Design review of the part built by this model. Coordinates are the model's own, in mm. Face numbers are marked on the shaded views. A direction names the side the tool comes from. Coordinates: 2 decimals unless noted, no trailing zeros. Write each loop counter-clockwise with the first axis right and the second up, starting at its lowest first coordinate (ties: lowest second). Pieces come first, ordered by that corner, then holes. Notation, with made-up numbers: (67, -27.75) -> (120, -27.75) arc R15 cw to (120, -22.75) -> close; hole circle Ø3 at (41, 48.5). An arc over 180 degrees is marked (long way). Return JSON: item names as keys, results as strings. Group by question number.
Autodesk Inventor part; units mm, degrees
ref_plane "FDT_PIRODACC_M1_XY" through (-9.9, 0, 0) normal (-1, 0, 0) x (0, 1, 0)
ref_plane "FDT_PIRODACC_M1_YZ" through (-9.9, 0, 0) normal (0, 1, 0) x (0, 0, -1)
ref_plane "FDT_PIRODACC_M1_ZX" through (-9.9, 0, 0) normal (0, 0, -1) x (-1, 0, 0)
sketch "Sketch_1" plane through (0, 0, 0) normal (0, 0, 1) x (1, 0, 0)
  line L0 (38, 0) -> (-4.2, 0)
  line L1 (-4.2, 0) -> (-4.2, 3)
  line L2 (-4.2, 3) -> (38, 3)
  line L3 (38, 3) -> (38, 0)
  line L4 (38, 0) -> (-4.2, 0)
revolve "Revolution1" add sketch "Sketch_1" angle 360 about axis through (38, 0, 0) along (1, 0, 0)
sketch "Sketch_11" plane through (0, 0, 0) normal (0, 0, 1) x (1, 0, 0)
  line L0 (38, 0) -> (35, 0)
  line L1 (35, 0) -> (35, 6)
  line L2 (35, 6) -> (38, 6)
  line L3 (38, 6) -> (38, 0)
  line L4 (38, 0) -> (35, 0)
revolve "Revolution2" add sketch "Sketch_11" angle 360 about axis through (38, 0, 0) along (1, 0, 0)
sketch "Sketch_19" plane through (0, 0, 0) normal (0, 0, 1) x (1, 0, 0)
  line L0 (-3.2, 0) -> (-14.2, 0)
  line L1 (-14.2, 0) -> (-14.2, 2.0095)
  line L2 (-14.2, 2.0095) -> (-13.7095, 2.5)
  line L3 (-13.7095, 2.5) -> (-6.7485, 2.5)
  line L4 (-6.7485, 2.5) -> (-5.1663, 1.9241)
  arc A0 (-5.1663, 1.9241) -> (-5.0295, 1.9) centre (-5.0295, 2.3) ccw
  line L5 (-5.0295, 1.9) -> (-4.6, 1.9)
  arc A1 (-4.6, 1.9) -> (-4.2, 2.3) centre (-4.6, 2.3) ccw
  line L6 (-4.2, 2.3) -> (-4.2, 2.5)
  line L7 (-4.2, 2.5) -> (-3.2, 2.5)
  line L8 (-3.2, 2.5) -> (-3.2, 0)
  line L9 (-3.2, 0) -> (-14.2, 0)
revolve "Revolution3" add sketch "Sketch_19" angle 360 about axis through (-3.2, 0, 0) along (1, 0, 0)
thread "Thread1"
sketch "Sketch_20" plane through (0, 0, 0) normal (0, 0, 1) x (1, 0, 0)
  line L0 (-23.4, -10.5) -> (3.1188, -10.5)
  line L1 (3.1188, -10.5) -> (-1.5, -2.5)
  line L2 (-1.5, -2.5) -> (-4.2, -2.5)
  line L3 (-4.2, -2.5) -> (-4.2, -7.5)
  line L4 (-4.2, -7.5) -> (-19.2, -7.5)
  line L5 (-19.2, -7.5) -> (-19.2, 7.5)
  line L6 (-19.2, 7.5) -> (-4.2, 7.5)
  line L7 (-4.2, 7.5) -> (-4.2, 2.5)
  line L8 (-4.2, 2.5) -> (-1.5, 2.5)
  line L9 (-1.5, 2.5) -> (3.1188, 10.5)
  line L10 (3.1188, 10.5) -> (-23.4, 10.5)
  line L11 (-23.4, 10.5) -> (-23.4, -10.5)
extrude "Extrusion1" cut sketch "Sketch_20" along normal mid plane 12
ref_plane "FDT_PIRODACC_M1_XY" through (-9.9, 0, 0) normal (-1, 0, 0) x (0, 1, 0)
ref_plane "FDT_PIRODACC_M1_YZ" through (-9.9, 0, 0) normal (0, 1, 0) x (0, 0, -1)
ref_plane "FDT_PIRODACC_M1_ZX" through (-9.9, 0, 0) normal (0, 0, -1) x (-1, 0, 0)
ref_plane "NUT1_XY" through (-8.55, 0, 0) normal (1, 0, 0) x (0, 0, -1)
ref_plane "NUT1_YZ" through (-8.55, 0, 0) normal (0, 0, -1) x (0, 1, 0)
ref_plane "NUT1_ZX" through (-8.55, 0, 0) normal (0, 1, 0) x (1, 0, 0)
ref_plane "PISTON_XY" through (38, 0, 0) normal (1, 0, 0) x (0, 0, -1)
ref_plane "PISTON_YZ" through (38, 0, 0) normal (0, 0, -1) x (0, 1, 0)
ref_plane "PISTON_ZX" through (38, 0, 0) normal (0, 1, 0) x (1, 0, 0)
properties part number "536203 ADN-15-P-A_(KS)"
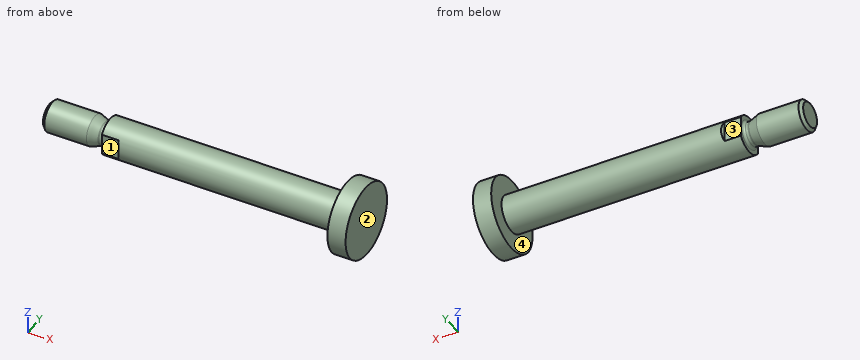
Q1. For P1, Ø3, axis at x = 19, y = 3, coming from the +Z side; P2, Ø0.8, axis at x = -2, z = -0.5, coming from the +Y side; P3, Ø5, axis at x = -2, z = -0.5, coming from the +Y side, all flat-tipped, find the tip position at first contact; note any pin that passes through.
Q2. Wall thickness on L1, parallel to Y at x = 23, z = -0.25; L2, parallel to X at y = -2.5, z = 3.75; L3, parallel to X at y = -1.75, z = -2.25: over which ranges is each line inside the solid? List them lowest first.
Q3. We need section A-A on y = 0. Write out the cut boundary in (x, z).
Q4. For the marked faces 1, 2, 3 and 4, list the 3-axis set-ups (+Z, -Z, +X, -X, +Y, -Y) from which the entire face can be reached by the end or side of a thin tool; tool diameter is ignored.
Q5. We need section D-D on z = -5. Write out the cut boundary in (x, y).
Q6. We need section B-B on z = 0. Write out the cut boundary in (x, y).
Q7. We need section C-C on x = 0. Write out the cut boundary in (y, z), plus the area to 3 significant figures.
Findings below:
{
 "1": {"P1": "stops at z = 2.6", "P2": "stops at y = 2.5", "P3": "stops at y = 3"},
 "2": {"L1": "y = -2.99 to 2.99", "L2": "x = 35 to 38", "L3": "x = -4.2 to 38"},
 "3": {"outline": "(-14.2, -2.01) -> (-13.71, -2.5) -> (-6.75, -2.5) -> (-5.17, -1.92) arc R0.4 cw to (-5.03, -1.9) -> (-4.6, -1.9) arc R0.4 cw to (-4.2, -2.3) -> (-4.2, -3) -> (35, -3) -> (35, -6) -> (38, -6) -> (38, 6) -> (35, 6) -> (35, 3) -> (-4.2, 3) -> (-4.2, 2.3) arc R0.4 cw to (-4.6, 1.9) -> (-5.03, 1.9) arc R0.4 cw to (-5.17, 1.92) -> (-6.75, 2.5) -> (-13.71, 2.5) -> (-14.2, 2.01) -> close"},
 "4": {"face 1": "+Z, -Z, -X, -Y", "face 2": "+Z, -Z, +X, +Y, -Y", "face 3": "+Z, -Z, -X, +Y", "face 4": "-X"},
 "5": {"outline": "(35, -3.32) -> (38, -3.32) -> (38, 3.32) -> (35, 3.32) -> close"},
 "6": {"outline": "(-14.2, -2.01) -> (-13.71, -2.5) -> (-6.75, -2.5) -> (-5.17, -1.92) arc R0.4 cw to (-5.03, -1.9) -> (-4.6, -1.9) arc R0.4 cw to (-4.2, -2.3) -> (-4.2, -2.5) -> (-1.5, -2.5) -> (-1.21, -3) -> (35, -3) -> (35, -6) -> (38, -6) -> (38, 6) -> (35, 6) -> (35, 3) -> (-1.21, 3) -> (-1.5, 2.5) -> (-4.2, 2.5) -> (-4.2, 2.3) arc R0.4 cw to (-4.6, 1.9) -> (-5.03, 1.9) arc R0.4 cw to (-5.17, 1.92) -> (-6.75, 2.5) -> (-13.71, 2.5) -> (-14.2, 2.01) -> close"},
 "7": {"outline": "circle Ø6 at (0, 0)", "area": "28.3 mm^2"}
}
